```python
from build123d import *

# Parameters (mm, degrees)
ESQUISSE1_W                         = 45
ESQUISSE1_H                         = 35
BOSS_EXTRU_1_DEPTH                  = 35
ESQUISSE2_R                         = 10
ENL_V_MAT_EXTRU_1_DEPTH             = 10
ESQUISSE3_W                         = 35
ESQUISSE3_H                         = 35
ENL_V_MAT_EXTRU_2_DEPTH             = 30
ESQUISSE4_R                         = 6.5
ENL_V_MAT_EXTRU_3_DEPTH             = 60.634302209
ESQUISSE15_W                        = 35
ESQUISSE15_H                        = 1.5
BOSS_EXTRU_2_DEPTH                  = 30
CONG_1_R                            = 5
DIAM_TRE_DU_PER_AGE_3_2_3_2_1_D     = 3.2
DIAM_TRE_DU_PER_AGE_3_2_3_2_1_DEPTH = 7
TROU_TARAUD_M3X0_52_D               = 2.5
TROU_TARAUD_M3X0_52_DEPTH           = 6.5
TROU_TARAUD_M3X0_52_TIP             = 0.751075774
TROU_TARAUD_M3X0_53_D               = 2.5
TROU_TARAUD_M3X0_53_DEPTH           = 6.5
TROU_TARAUD_M3X0_53_TIP             = 0.751075774
TROU_TARAUD_M3X0_54_D               = 2.5
TROU_TARAUD_M3X0_54_DEPTH           = 6.5
TROU_TARAUD_M3X0_54_TIP             = 0.751075774
TROU_TARAUD_M3X0_56_D               = 2.5
TROU_TARAUD_M3X0_56_DEPTH           = 6.5
TROU_TARAUD_M3X0_56_TIP             = 0.751075774
TROU_TARAUD_M3X0_57_D               = 2.5


with BuildPart() as part:
    # Esquisse1 → Boss.-Extru.1 (new body)
    with BuildSketch(Plane.XY):
        Rectangle(ESQUISSE1_W, ESQUISSE1_H)
    extrude(amount=BOSS_EXTRU_1_DEPTH)

    # Esquisse2 → Enlèv. mat.-Extru.1 (cut)
    with BuildSketch(Plane(origin=(0, 17.5, 0), x_dir=(1, 0, 0), z_dir=(0, 1, 0))):
        with Locations(Location((1.5, -17.5, 0), (0, 0, 270))):
            Circle(ESQUISSE2_R)
    extrude(amount=-ENL_V_MAT_EXTRU_1_DEPTH, mode=Mode.SUBTRACT)

    # Esquisse3 → Enlèv. mat.-Extru.2 (cut)
    with BuildSketch(Plane.XZ.offset(17.5)):
        with Locations((0, 17.5)):
            Rectangle(ESQUISSE3_W, ESQUISSE3_H)
    extrude(amount=-ENL_V_MAT_EXTRU_2_DEPTH, mode=Mode.SUBTRACT)

    # Esquisse4 → Enlèv. mat.-Extru.3 (cut, through all)
    with BuildSketch(Plane.ZY.offset(22.5)):
        with Locations((17.5, -7.5)):
            Circle(ESQUISSE4_R)
    extrude(amount=-ENL_V_MAT_EXTRU_3_DEPTH, mode=Mode.SUBTRACT)

    # Esquisse15 → Boss.-Extru.2 (add)
    with BuildSketch(Plane.XZ.offset(-12.5)):
        with Locations((0, 34.25)):
            Rectangle(ESQUISSE15_W, ESQUISSE15_H)
        with Locations((0, 0.75)):
            Rectangle(ESQUISSE15_W, ESQUISSE15_H)
    extrude(amount=BOSS_EXTRU_2_DEPTH)

    # Congé1
    cong_1_edges = [part.edges().sort_by_distance(p)[0] for p in [
        (17.5, -2.5, 33.5),
        (-17.5, -2.5, 33.5),
        (17.5, -2.5, 1.5),
        (-17.5, -2.5, 1.5),
    ]]
    fillet(cong_1_edges, radius=CONG_1_R)

    # Diamètre du perçage Ø3.2 (3.2)1
    with Locations(Plane(origin=(0, 12.5, 0), x_dir=(-1, 0, 0), z_dir=(0, -1, 0))):
        with Locations((-14.5, -17.5), (-1.5, -4.5), (11.5, -17.5), (-1.5, -30.5)):
            Hole(DIAM_TRE_DU_PER_AGE_3_2_3_2_1_D / 2, depth=DIAM_TRE_DU_PER_AGE_3_2_3_2_1_DEPTH)

    # Trou taraudé M3x0.52
    with Locations(Plane(origin=(0, -17.5, 0), x_dir=(-1, 0, 0), z_dir=(0, -1, 0))):
        with Locations((-20, -7.5), (20, -27.5), (-20, -27.5), (20, -7.5)):
            Hole(TROU_TARAUD_M3X0_52_D / 2, depth=TROU_TARAUD_M3X0_52_DEPTH)
            with Locations((0, 0, -(TROU_TARAUD_M3X0_52_DEPTH + TROU_TARAUD_M3X0_52_TIP / 2))):  # 118° drill point
                Cone(0, TROU_TARAUD_M3X0_52_D / 2, TROU_TARAUD_M3X0_52_TIP, mode=Mode.SUBTRACT)

    # Trou taraudé M3x0.53
    with Locations(Plane(origin=(0, 0, 0), x_dir=(-1, 0, 0), z_dir=(0, 0, -1))):
        with Locations((-20, 8.5), (20, -11.5), (-20, -11.5), (20, 8.5)):
            Hole(TROU_TARAUD_M3X0_53_D / 2, depth=TROU_TARAUD_M3X0_53_DEPTH)
            with Locations((0, 0, -(TROU_TARAUD_M3X0_53_DEPTH + TROU_TARAUD_M3X0_53_TIP / 2))):  # 118° drill point
                Cone(0, TROU_TARAUD_M3X0_53_D / 2, TROU_TARAUD_M3X0_53_TIP, mode=Mode.SUBTRACT)

    # Trou taraudé M3x0.54
    with Locations(Plane.XY.offset(35)):
        with Locations((20, 8.5), (-20, 8.5), (20, -11.5), (-20, -11.5)):
            Hole(TROU_TARAUD_M3X0_54_D / 2, depth=TROU_TARAUD_M3X0_54_DEPTH)
            with Locations((0, 0, -(TROU_TARAUD_M3X0_54_DEPTH + TROU_TARAUD_M3X0_54_TIP / 2))):  # 118° drill point
                Cone(0, TROU_TARAUD_M3X0_54_D / 2, TROU_TARAUD_M3X0_54_TIP, mode=Mode.SUBTRACT)

    # Trou taraudé M3x0.56
    with Locations(Plane(origin=(22.5, 0, 0), x_dir=(0, 0, -1), z_dir=(1, 0, 0))):
        with Locations((-27.5, -7.5), (-7.5, 4.5), (-27.5, 4.5), (-7.5, -7.5)):
            Hole(TROU_TARAUD_M3X0_56_D / 2, depth=TROU_TARAUD_M3X0_56_DEPTH)
            with Locations((0, 0, -(TROU_TARAUD_M3X0_56_DEPTH + TROU_TARAUD_M3X0_56_TIP / 2))):  # 118° drill point
                Cone(0, TROU_TARAUD_M3X0_56_D / 2, TROU_TARAUD_M3X0_56_TIP, mode=Mode.SUBTRACT)

    # Trou taraudé M3x0.57 (through all)
    with Locations(Plane(origin=(0, 12.5, 0), x_dir=(-1, 0, 0), z_dir=(0, -1, 0))):
        with Locations((-12.5, -28.5), (12.5, -6.5), (-12.5, -6.5), (12.5, -28.5)):
            Hole(TROU_TARAUD_M3X0_57_D / 2)


solid = part.part
```
CAD build for the part. Positions are in the model's coordinates, mm. A direction names the side the tool comes from. Give positions to 0.01 mm unless a question says otherwise; leave off trailing zeros. Order: outer loops, then holes, each group sorted by start corner. A loop starts at its lowest first (then second) coordinate and runs counter-clockwise, first axis right, second up. Notation, with made-up numbers: M -4,-37 L 3,-37 A28 cw 3,-3 Z; hole C -3,34 d8. An arc over 180 degrees is marked long. Put each result on its own line as item: value. Start each with the question number.
(1) Saw through at A-A, the plane y = -5. Write the cut outline in (x, z), then the cut area to 3 significant figures.
(2) Saw through at C-C, the plane x = 10.5. Write the cut outline in (y, z).
(3) Saw through at D-D, the plane z = 4.5. Write the cut outline in (x, y), then the cut area to 3 significant figures.
(4) Mould opens along Z. For faces 5 (the cylindrical face through (-18.81, -11.12, 3.3)), 6 (the flat face through (0, 0, 0)), 7 (the flat face through (0, -2, 1.5)) say: +Z half, -Z half, draft (parallel to the pull), parting line (faces both ways), or undercut.
(5) Flat gauge pins, fed straight in: pin 1 Ø6 at (x, z) = (-8, 22.5) entering from -Y; pin 2 Ø3 at (x, y) = (20, 8.5) entering from +Z; pin 3 Ø1.5 at (y, z) = (-7.5, 27.5) entering from +X; pin 4 Ø2 at (x, z) = (20, 7.5) entering from -Y. Where does each tip first touch, or does it go through?
(6) Drill centre lines: line 1 along X through (y, z) = (13.8, 6.5); line 2 along Z through (x, y) = (12.5, 14.6); line 3 along X through (y, z) = (-11, 33). Where is each one in solid material? Low to high.
(7) Saw through at B-B, the plane z = 17.5. Write the cut outline in (x, y), then the cut area to 3 significant figures.
(8) Which spindle directions (+Z, -Z, +X, -X, +Y, -Y) get a long thin tool onto all of the face, cutting with end or side? Do faces 1 (the flat face through (-8, 12.5, 21.3)), 2 (the cylindrical face through (-18.81, 8.88, 3.3)), 3 (the cylindrical face through (18.81, -11.12, 31.7)), 4 (the cylindrical face through (13.32, 15.04, 16.42)). Say none if no direction does.
Check result:
1. outline: M -22.5,0 L 22.5,0 L 22.5,11.5 L 17.5,11.5 L 17.5,6.5 A5 cw 12.5,1.5 L -12.5,1.5 A5 cw -17.5,6.5 L -17.5,11.5 L -22.5,11.5 Z; M -22.5,23.5 L -17.5,23.5 L -17.5,28.5 A5 cw -12.5,33.5 L 12.5,33.5 A5 cw 17.5,28.5 L 17.5,23.5 L 22.5,23.5 L 22.5,35 L -22.5,35 Z
1. area: 356 mm2
2. outline: M -17.5,0 L 17.5,0 L 17.5,13.14 L 12.5,13.14 L 12.5,1.5 L -17.5,1.5 Z; M -17.5,33.5 L 12.5,33.5 L 12.5,21.86 L 17.5,21.86 L 17.5,35 L -17.5,35 Z
3. outline: M -22.5,-17.5 L -17.08,-17.5 L -17.08,12.5 L -0.1,12.5 L -0.1,17.5 L -22.5,17.5 Z; M 3.1,12.5 L 17.08,12.5 L 17.08,-17.5 L 22.5,-17.5 L 22.5,17.5 L 3.1,17.5 Z; hole C -20,-11.5 d2.5; hole C -20,8.5 d2.5; hole C 20,-11.5 d2.5; hole C 20,8.5 d2.5
3. area: 514 mm2
4. face 5: draft
4. face 6: -Z half
4. face 7: undercut
5. pin 1: stops at y = 12.5
5. pin 2: stops at z = 35
5. pin 3: stops at x = -17.5
5. pin 4: stops at y = -10.85
6. line 1: x = -22.5 to -13.75, -11.25 to 11.25, 13.75 to 22.5
6. line 2: z = 0 to 5.25, 7.75 to 27.25, 29.75 to 35
6. line 3: x = -22.5 to -21.15, -18.85 to -14.68, 14.68 to 18.85, 21.15 to 22.5
7. outline: M -22.5,-17.5 L -17.5,-17.5 L -17.5,-14 L -22.5,-14 Z; M -22.5,-1 L -17.5,-1 L -17.5,12.5 L -13.1,12.5 L -13.1,17.5 L -22.5,17.5 Z; M -9.9,12.5 L -8.5,12.5 L -8.5,17.5 L -9.9,17.5 Z; M 11.5,12.5 L 12.9,12.5 L 12.9,17.5 L 11.5,17.5 Z; M 16.1,12.5 L 17.5,12.5 L 17.5,-1 L 22.5,-1 L 22.5,17.5 L 16.1,17.5 Z; M 17.5,-17.5 L 22.5,-17.5 L 22.5,-14 L 17.5,-14 Z
7. area: 263 mm2
8. face 1: -Y
8. face 2: -Z
8. face 3: +Z
8. face 4: +Y, -Y
